```python
from build123d import *

# Parameters (mm, degrees)
EXTRUDE_1_DEPTH     = 10.5
SKETCH_2_R          = 2.25
CUT_EXTRUDE_1_DEPTH = 4
SKETCH_3_R          = 2.75
SKETCH_3_R_2        = 2.25
EXTRUDE_2_DEPTH     = 0.5
CHAMFER_1_SIZE      = 0.25
SKETCH_4_R          = 3.5
EXTRUDE_3_DEPTH     = 8.5
DRAFT_1_ANGLE       = 5


with BuildPart() as part:
    # 草图1 → 凸台-拉伸1 (new body)
    with BuildSketch(Plane(origin=(0, 0, 0), x_dir=(1, 0, 0), z_dir=(0, 1, 0))):
        with BuildLine():
            Line((-28, 20), (28, 20))
            ThreePointArc((28, 20), (29.414213562, 19.414213562), (30, 18))
            Line((30, 18), (30, -18))
            ThreePointArc((30, -18), (29.414213562, -19.414213562), (28, -20))
            Line((28, -20), (-28, -20))
            ThreePointArc((-28, -20), (-29.414213562, -19.414213562), (-30, -18))
            Line((-30, -18), (-30, 18))
            ThreePointArc((-30, 18), (-29.414213562, 19.414213562), (-28, 20))
        make_face()
    extrude(amount=EXTRUDE_1_DEPTH)

    # 草图2 → 切除-拉伸1 (cut)
    with BuildSketch(Plane(origin=(0, 0, -20), x_dir=(-1, 0, 0), z_dir=(0, 0, -1))):
        with Locations((-18, 4)):
            Circle(SKETCH_2_R)
        with Locations((-12, 4)):
            Circle(SKETCH_2_R)
        with Locations((-6, 4)):
            Circle(SKETCH_2_R)
    extrude(amount=-CUT_EXTRUDE_1_DEPTH, mode=Mode.SUBTRACT)

    # 草图3 → 凸台-拉伸2 (add)
    with BuildSketch(Plane(origin=(0, 0, -20), x_dir=(-1, 0, 0), z_dir=(0, 0, -1))):
        with Locations((-18, 4)):
            Circle(SKETCH_3_R)
        with Locations((-18, 4)):
            Circle(SKETCH_3_R_2, mode=Mode.SUBTRACT)
        with Locations((-12, 4)):
            Circle(SKETCH_3_R)
        with Locations((-12, 4)):
            Circle(SKETCH_3_R_2, mode=Mode.SUBTRACT)
        with Locations((-6, 4)):
            Circle(SKETCH_3_R)
        with Locations((-6, 4)):
            Circle(SKETCH_3_R_2, mode=Mode.SUBTRACT)
    extrude(amount=EXTRUDE_2_DEPTH)

    # 倒角1
    chamfer_1_edges = [part.edges().sort_by_distance(p)[0] for p in [
        (20.75, 4, -20.5),
        (14.75, 4, -20.5),
        (8.75, 4, -20.5),
    ]]
    chamfer(chamfer_1_edges, length=CHAMFER_1_SIZE)

    # 草图4 → 凸台-拉伸3 (add)
    with BuildSketch(Plane.XY.offset(20)):
        with Locations((13, 5.25)):
            Circle(SKETCH_4_R)
    extrude(amount=EXTRUDE_3_DEPTH)

    # 拔模1
    draft_1_faces = [part.faces().sort_by_distance(p)[0] for p in [
        (9.5, 5.25, 24.25),
    ]]
    draft(draft_1_faces, Plane(origin=(13, 5.25, 28.5), x_dir=(1, 0, 0), z_dir=(0, 0, 1)), DRAFT_1_ANGLE)


solid = part.part
```
The model under review builds one solid part; all positions refer to its coordinate system, in mm. A direction names the side the tool comes from. Round coordinates to 2 decimals unless told otherwise and drop trailing zeros. Order: outer loops, then holes, each group sorted by start corner. A loop starts at its lowest first (then second) coordinate and runs counter-clockwise, first axis right, second up. Notation, with made-up numbers: M -13,46 L 2,46 A19 ccw 2,65 Z; hole C 30.5,-13 d3. An arc over 180 degrees is marked long. Use a Markdown table: item, result.
1) Consider section A-A (z = -17). Write out the cut boundary in (x, y).
Report:
| item | result |
|---|---|
| outline | M -30,0 L 30,0 L 30,10.5 L -30,10.5 Z; hole C 6,4 d4.5; hole C 12,4 d4.5; hole C 18,4 d4.5 |
2) Wall thickness on line 1 along Y through (x, z) = (6, -19); line 2 along Z through (x, y) = (-14.5, 1.5); line 3 along Z through (x, y) = (6.5, 2.25): over which ranges is each line inside the solid? List them lowest first. Write a range as [from, to].
Report:
| item | result |
|---|---|
| line 1 | [0, 1.75], [6.25, 10.5] |
| line 2 | [-20, 20] |
| line 3 | [-16, 20] |
3) Draft analysis for pull direction X (two halves, no side actions). For faces 1 (the face through (6, 4, -16)), 2 (the face through (0, 5, 20)), 3 (the face through (9.923, 2.891, 24.19)), state which applies: released by +X, released by -X, zero draft, split by the parting line, or undercut.
Report:
| item | result |
|---|---|
| face 1 | undercut |
| face 2 | zero draft |
| face 3 | split by the parting line |
4) Tool access review of faces 4 (the face through (-29.43, 5.18, -19.4)), 5 (the face through (12, 4, -16)): name each direction out of +Z, -Z, +X, -X, +Y, -Y from which nothing blocks a thin tool from reaching the whole face with its end or side.
Report:
| item | result |
|---|---|
| face 4 | -Z, -X, +Y, -Y |
| face 5 | -Z |
5) Consider section C-C (z = 24.5). Write out the cut boundary in (x, y), then the cut area to 3 significant figures.
Report:
| item | result |
|---|---|
| outline | C 13,5.25 d7.7 |
| area | 46.6 mm^2 |
6) Consider section B-B (x = 2.5). Write out the cut boundary in (y, z), then the cut area to 3 significant figures.
Report:
| item | result |
|---|---|
| outline | M 0,-20 L 10.5,-20 L 10.5,20 L 0,20 Z |
| area | 420 mm^2 |
7) Insertion check: pin 1 (4 mm diameter, centred on x = -24, y = 5, fed in from +Z); pin 2 (1.3 mm diameter, centred on x = 6.5, y = 3.5, fed in from -Z). Each pin has a flat end and moves straight along its axis. Give the tip position at first contact, or say it passes through.
Report:
| item | result |
|---|---|
| pin 1 | z = 20 |
| pin 2 | z = -16 |
